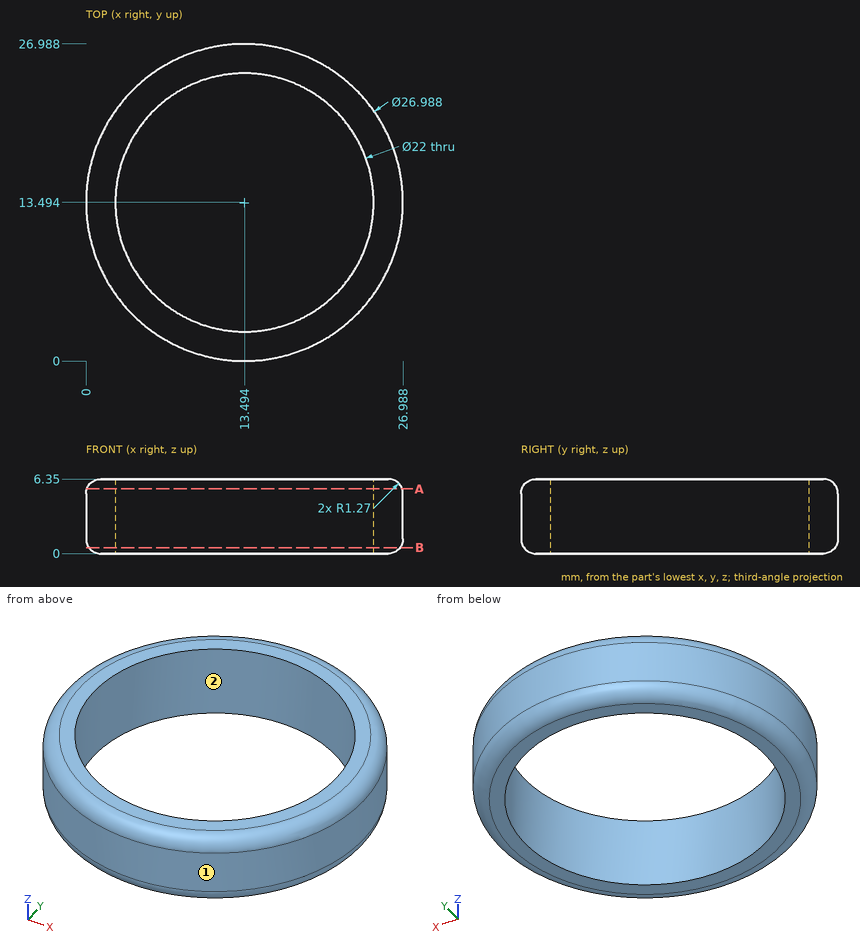
Input: dimensioned drawing with shaded views. Units: mm. Origin: part minimum x, y, z. Give positions to 0.01 mm unless a question says otherwise; leave off trailing zeros. Loops run counter-clockwise (first coordinate to the right, second up) from the corner with the lowest first, then second, coordinate; pieces in that order, holes last. Notation, with made-up numbers: M -17,72 L 8,72 A21 cw 8,88 Z; hole C -10,55.5 d2. An arc over 180 degrees is marked long. Put each result on its own line as item: value.
1) First-contact query: P1, Ø1.5, axis at x = 4.5, z = 5, coming from the -Y side; P2, Ø13, axis at x = 13.49, y = 13.49, coming from the +Z side (3 decimals); P3, Ø2, axis at y = 18, z = 4.5, coming from the +X side. Flat tips, straight axial feed; report the tip coordinate or a pass-through.
Computed values:
P1: stops at y = 2.81
P2: passes through
P3: stops at x = 26.52
2) Mould query, pull axis X, two halves, no side actions, for the marked faces 1 and 2. Classes: released by +X, released by -X, zero draft, split by the parting line, or undercut.
Computed values:
face 1: split by the parting line
face 2: undercut
3) Material intervals for L1, parallel to X at y = 17, z = 3 (1 decimal); L2, parallel to X at y = 12.25, z = 3 (1 decimal); L3, parallel to Y at x = 7.5, z = 3.25 (1 decimal), sorted ascending. Write a range as from..to.
Computed values:
L1: x = 0.5..3.1, 23.9..26.5
L2: x = 0.1..2.6, 24.4..26.9
L3: y = 1.4..4.3, 22.7..25.6
4) Cut plane A-A, the plane z = 5.5. Return the cut outline in (x, y) (1 decimal), plus the area to 3 significant figures.
Computed values:
outline: C 13.5,13.5 d26.8; hole C 13.5,13.5 d22
area: 186 mm^2
5) Cut plane B-B, the plane z = 0.5. Return the cut outline in (x, y).
Computed values:
outline: C 13.49,13.49 d26.47; hole C 13.49,13.49 d22
